from build123d import *

# Parameters (mm, degrees)
EXTRUDE_1_DEPTH     = 3
SKETCH_2_R          = 1.5
CUT_EXTRUDE_1_DEPTH = 3


with BuildPart() as part:
    # 草图1 → 凸台-拉伸1 (new body)
    with BuildSketch(Plane(origin=(0, 0, 0), x_dir=(1, 0, 0), z_dir=(0, 1, 0))):
        with BuildLine():
            Line((0, 0), (25, 0))
            Line((25, 0), (45, -28))
            Line((45, -28), (45, -43))
            Line((45, -43), (30, -43))
            Line((30, -43), (30, -38.679491924))
            ThreePointArc((30, -38.679491924), (29.659258263, -36.091301473), (28.660254038, -33.679491924))
            Line((28.660254038, -33.679491924), (22.386751346, -22.813466521))
            ThreePointArc((22.386751346, -22.813466521), (18.726497308, -19.153212483), (13.726497308, -17.813466521))
            Line((13.726497308, -17.813466521), (11.273502692, -17.813466521))
            ThreePointArc((11.273502692, -17.813466521), (6.273502692, -19.153212483), (2.613248654, -22.813466521))
            Line((2.613248654, -22.813466521), (-3.660254038, -33.679491924))
            ThreePointArc((-3.660254038, -33.679491924), (-4.659258263, -36.091301473), (-5, -38.679491924))
            Line((-5, -38.679491924), (-5, -43))
            Line((-5, -43), (-20, -43))
            Line((-20, -43), (-20, -28))
            Line((-20, -28), (0, 0))
        make_face()
    extrude(amount=EXTRUDE_1_DEPTH)

    # 草图2 → 切除-拉伸1 (cut)
    with BuildSketch(Plane(origin=(0, 3, 0), x_dir=(1, 0, 0), z_dir=(0, 1, 0))):
        with Locations(Location((-12.5, -34, 0), (0, 0, 270))):
            Circle(SKETCH_2_R)
        with Locations(Location((37.5, -34, 0), (0, 0, 270))):
            Circle(SKETCH_2_R)
        with Locations(Location((3.5, -7.5, 0), (0, 0, 270))):
            Circle(SKETCH_2_R)
        with Locations(Location((21.5, -7.5, 0), (0, 0, 270))):
            Circle(SKETCH_2_R)
    extrude(amount=-CUT_EXTRUDE_1_DEPTH, mode=Mode.SUBTRACT)


solid = part.part
CAD build for the part. Positions are in the model's coordinates, mm. A direction names the side the tool comes from. Coordinates: 2 decimals unless noted, no trailing zeros. Order: outer loops, then holes, each group sorted by start corner. A loop starts at its lowest first (then second) coordinate and runs counter-clockwise, first axis right, second up. Notation, with made-up numbers: (15.25, 38.25) -> (22.25, 38.25) arc R27 ccw to (22.25, 67.25) -> close; hole circle Ø4 at (62, -1.5). An arc over 180 degrees is marked (long way). Answer in a Markdown table with one row per item.
1) Flat gauge pins, fed straight in: P1, Ø1.8, axis at x = 37.5, z = 34, coming from the -Y side; P2, Ø1.5, axis at y = 2, z = 19.5, coming from the +X side. Where does each tip first touch, or does it go through?
Check values:
| item | result |
|---|---|
| P1 | through |
| P2 | x = 39.46 |
2) Band-saw the part on C-C (y = 0.65). List the corners of the cut face in (x, z), and give its area (3 significant figures).
Check values:
| item | result |
|---|---|
| outline | (-20, 28) -> (0, 0) -> (25, 0) -> (45, 28) -> (45, 43) -> (30, 43) -> (30, 38.68) arc R10 cw to (28.66, 33.68) -> (22.39, 22.81) arc R10 cw to (13.73, 17.81) -> (11.27, 17.81) arc R10 cw to (2.61, 22.81) -> (-3.66, 33.68) arc R10 cw to (-5, 38.68) -> (-5, 43) -> (-20, 43) -> close; hole circle Ø3 at (-12.5, 34); hole circle Ø3 at (3.5, 7.5); hole circle Ø3 at (21.5, 7.5); hole circle Ø3 at (37.5, 34) |
| area | 1,530 mm2 |
3) Mould opens along Z. For faces 1 (the face through (13, 3, 16)), 2 (the face through (-0.48, 1.48, 28.17)), 3 (the face through (22.51, 1.52, 6.39)) say: pulls with the +Z half, pulls with the -Z half, needs draft (parallel to the pull), parting line crosses it, or undercut.
Check values:
| item | result |
|---|---|
| face 1 | needs draft |
| face 2 | pulls with the +Z half |
| face 3 | undercut |
4) Drill centre lines: line 1 (X direction, y = 1, z = 7.5); line 2 (X direction, y = 1.45, z = 35); line 3 (X direction, y = 2.3, z = 34). Where is each one in solid material? Low to high.
Check values:
| item | result |
|---|---|
| line 1 | -5.36 to 2, 5 to 20, 23 to 30.36 |
| line 2 | -20 to -13.62, -11.38 to -4.3, 29.3 to 36.38, 38.62 to 45 |
| line 3 | -20 to -14, -11 to -3.84, 28.84 to 36, 39 to 45 |
5) Band-saw the part on B-B (z = 30). List the corners of the cut face in (x, y).
Check values:
| item | result |
|---|---|
| outline | (-20, 0) -> (-1.54, 0) -> (-1.54, 3) -> (-20, 3) -> close; (26.54, 0) -> (45, 0) -> (45, 3) -> (26.54, 3) -> close |
6) Band-saw the part on D-D (z = 7.5). List the corners of the cut face in (x, y).
Check values:
| item | result |
|---|---|
| outline | (-5.36, 0) -> (2, 0) -> (2, 3) -> (-5.36, 3) -> close; (5, 0) -> (20, 0) -> (20, 3) -> (5, 3) -> close; (23, 0) -> (30.36, 0) -> (30.36, 3) -> (23, 3) -> close |
7) Which spindle directions (+Z, -Z, +X, -X, +Y, -Y) get a long thin tool onto all of the face, cutting with end or side? Do faces 4 (the face through (12, 1, 0)), 5 (the face through (29.67, 1.48, 36.13)). Say none if no direction does.
Check values:
| item | result |
|---|---|
| face 4 | -Z, +X, -X, +Y, -Y |
| face 5 | +Z, +Y, -Y |
8) Band-saw the part on A-A (x = -12.5). List the corners of the cut face in (y, z), and give its area (3 significant figures).
Check values:
| item | result |
|---|---|
| outline | (0, 17.5) -> (3, 17.5) -> (3, 32.5) -> (0, 32.5) -> close; (0, 35.5) -> (3, 35.5) -> (3, 43) -> (0, 43) -> close |
| area | 67.5 mm2 |
